```python
from build123d import *

# Parameters (mm, degrees)
SKETCH1_W           = 100
SKETCH1_H           = 65
BOSS_EXTRUDE1_DEPTH = 10
SKETCH2_R           = 2.5
CUT_EXTRUDE1_DEPTH  = 10
SKETCH3_R           = 2.5
CUT_EXTRUDE2_DEPTH  = 4


with BuildPart() as part:
    # Sketch1 → Boss-Extrude1 (new body)
    with BuildSketch(Plane(origin=(0, 0, 0), x_dir=(1, 0, 0), z_dir=(0, 1, 0))):
        with Locations((50, 32.5)):
            Rectangle(SKETCH1_W, SKETCH1_H)
    extrude(amount=BOSS_EXTRUDE1_DEPTH)

    # Sketch2 → Cut-Extrude1 (cut)
    with BuildSketch(Plane(origin=(0, 0, -65), x_dir=(-1, 0, 0), z_dir=(0, 0, -1))):
        with Locations((-59, 5)):
            Circle(SKETCH2_R)
        with Locations((-41, 5)):
            Circle(SKETCH2_R)
    extrude(amount=-CUT_EXTRUDE1_DEPTH, mode=Mode.SUBTRACT)

    # Sketch3 → Cut-Extrude2 (cut)
    with BuildSketch(Plane(origin=(0, 10, 0), x_dir=(1, 0, 0), z_dir=(0, 1, 0))):
        with Locations(Location((29.75, 3.575, 0), (0, 0, 270))):
            Circle(SKETCH3_R)
        with Locations(Location((70.25, 61.425, 0), (0, 0, 270))):
            Circle(SKETCH3_R)
    extrude(amount=-CUT_EXTRUDE2_DEPTH, mode=Mode.SUBTRACT)


solid = part.part
```
Geometry check sheet. Reference: the model listing, model coordinates, mm. A direction names the side the tool comes from. Give positions to 0.01 mm unless a question says otherwise; leave off trailing zeros. Order: outer loops, then holes, each group sorted by start corner. A loop starts at its lowest first (then second) coordinate and runs counter-clockwise, first axis right, second up.
1. Release check for a two-part mould opening along Y. For faces 4 (the face through (49, 0, -33)), 5 (the face through (32.23, 8.03, -3.9)), 6 (the face through (41, 5, -55)) record: pulls with the +Y half, pulls with the -Y half, needs draft (parallel to the pull), parting line crosses it, or undercut.
2. Section check A-A, the plane x = 70.25. Enter the section's corners in (y, z) (3 decimals).
3. Section check B-B, the plane y = 5. Enter the section's corners in (x, z), and give its area (3 significant figures).
4. Section check C-C, the plane x = 59. Enter the section's corners in (y, z), and give its area (3 significant figures).
5. Thickness scan on L1, parallel to Y at x = 59, z = -59.25. Record the ranges inside material, lowest first.
6. Access from +Z, -Z, +X, -X, +Y, -Y to the whole of each face (thin tool, end or side, straight path). Record for faces 1 (the face through (100, 5, -32)), 2 (the face through (38.69, 4.04, -60.07)), 3 (the face through (70, 6, -61)).
7. Gauge pin test, flat ends, axial feed: pin 1 Ø2.5 at (x, z) = (29, -4.5) entering from +Y; pin 2 Ø1.5 at (x, y) = (41.5, 5) entering from -Z. Record the tip position at first contact, or that the pin passes through.
Values follow:
1. face 4: pulls with the -Y half
1. face 5: needs draft
1. face 6: undercut
2. outline: (0, -65) - (10, -65) - (10, -63.925) - (6, -63.925) - (6, -58.925) - (10, -58.925) - (10, 0) - (0, 0) - close
3. outline: (0, -65) - (38.5, -65) - (38.5, -55) - (43.5, -55) - (43.5, -65) - (56.5, -65) - (56.5, -55) - (61.5, -55) - (61.5, -65) - (100, -65) - (100, 0) - (0, 0) - close
3. area: 6,400 mm2
4. outline: (0, -65) - (2.5, -65) - (2.5, -55) - (7.5, -55) - (7.5, -65) - (10, -65) - (10, 0) - (0, 0) - close
4. area: 600 mm2
5. L1: y = 0 to 2.5, 7.5 to 10
6. face 1: +Z, -Z, +X, +Y, -Y
6. face 2: -Z
6. face 3: +Y
7. pin 1: stops at y = 6
7. pin 2: stops at z = -55
